from build123d import *

# Parameters (mm, degrees)
PAD_DEPTH       = 10
POCKET_DEPTH    = 6
POCKET001_DEPTH = 6
POCKET002_DEPTH = 11
FILLET_R        = 1
FILLET001_R     = 10
FILLET002_R     = 9
FILLET003_R     = 1


with BuildPart() as part:
    # Sketch → Pad (new body)
    with BuildSketch(Plane.XY):
        Polygon((-65, 10), (-65, 5), (-60, 5), (-60, -5), (-75, -5), (-75, -35), (-50, -35), (-50, -5), (-30, -5), (-30, 0), (-35, 0), (-35, 5), (-30, 5), (-30, 10), (-45, 10), (-45, 5), (-40, 5), (-40, 0), (-55, 0), (-55, 5), (-50, 5), (-50, 10), align=None)
    extrude(amount=PAD_DEPTH)

    # Sketch001 (on Face24 of Pad) → Pocket (cut)
    with BuildSketch(Plane.XY.offset(10)):
        Polygon((0, 15), (-80, 15), (-80, -5), (-60, -5), (-60, -35), (-50, -35), (-50, -5), (0, -5), align=None)
    extrude(amount=-POCKET_DEPTH, mode=Mode.SUBTRACT)

    # Sketch002 (on Face27 of Pocket) → Pocket001 (cut)
    with BuildSketch(Plane.XY.offset(10)):
        Polygon((-80, -8.189183), (-60, -11), (-60, -31), (-80, -28.189183), align=None)
    extrude(amount=-POCKET001_DEPTH, mode=Mode.SUBTRACT)

    # Sketch003 (on Face29 of Pocket001) → Pocket002 (cut)
    with BuildSketch(Plane.XY.offset(10)):
        Polygon((-60, -35), (-80, -32.189183), (-80, -40), (-60, -40), align=None)
    extrude(amount=-POCKET002_DEPTH, mode=Mode.SUBTRACT)

    # Fillet
    fillet_edges = [part.edges().sort_by_distance(p)[0] for p in [
        (-65, 5, 2),
        (-45, 5, 2),
        (-45, 10, 2),
        (-65, 10, 2),
        (-50, 10, 2),
        (-30, 10, 2),
        (-50, 5, 2),
        (-30, 5, 2),
    ]]
    fillet(fillet_edges, radius=FILLET_R)

    # Fillet001
    fillet001_edges = [part.edges().sort_by_distance(p)[0] for p in [
        (-50, -5, 2),
    ]]
    fillet(fillet001_edges, radius=FILLET001_R)

    # Fillet002
    fillet002_edges = [part.edges().sort_by_distance(p)[0] for p in [
        (-50, -35, 2),
    ]]
    fillet(fillet002_edges, radius=FILLET002_R)

    # Fillet003
    fillet003_edges = [part.edges().sort_by_distance(p)[0] for p in [
        (-30, -5, 2),
        (-30, 0, 2),
    ]]
    fillet(fillet003_edges, radius=FILLET003_R)


solid = part.part
The model under review builds one solid part; all positions refer to its coordinate system, in mm. A direction names the side the tool comes from. Give positions to 0.01 mm unless a question says otherwise; leave off trailing zeros. Order: outer loops, then holes, each group sorted by start corner. A loop starts at its lowest first (then second) coordinate and runs counter-clockwise, first axis right, second up. Notation, with made-up numbers: M 8.5,84.25 L 62.5,84.25 A12 ccw 62.5,91.25 Z; hole C 22.25,77 d1. An arc over 180 degrees is marked long. Answer in a Markdown table with one row per item. Add a question column.
1. For pin 1 Ø2 at (y, z) = (-16.5, 3) entering from +X; pin 2 Ø2 at (y, z) = (-30, 3) entering from +X; pin 3 Ø4.5 at (x, z) = (-42, 2.5) entering from -Y, all flat-tipped, find the tip position at first contact; note any pin that passes through.
2. Add section A-A on z = 8.25. State the section outline as (x, y) points, plus the area to 3 significant figures.
3. Machinability: for faces 1 (the flat face through (-60, -33, 7)), 2 (the cylindrical face through (-30.285, 5.301, 2.028)), 3 (the flat face through (-50, 7, 2)), which of the approach directions +Z, -Z, +X, -X, +Y, -Y give a long, thin tool a straight path to every point of the face, cutting with its end or side? Answer none if there is none.
4. Add section B-B on y = 1.5. State the section outline as (x, z) points, plus the area to 3 significant figures.
5. Add section C-C on x = -62.5. State the section outline as (y, z) points, plus the area to 3 significant figures.
6. Mouldability with a two-part tool opening along Y and no side actions: class faces 4 (the flat face through (-45, 8, 2)), 5 (the cylindrical face through (-52.566, -32.294, 2.028)), 6 (the flat face through (-55, 2, 2)) as released by +Y, released by -Y, zero draft, split by the parting line, or undercut.
7. Add section D-D on y = -7. State the section outline as (x, z) points, plus the area to 3 significant figures.
8. To check wall thickness, follow line 1 along X through (y, z) = (1, 0.5); line 2 along Z through (x, y) = (-67, -12.5); line 3 along Y through (x, z) = (-62, 7). State the ranges of each line that lie inside material, in increasing order.
The answers:
| question | item | result |
|---|---|---|
| 1 | pin 1 | x = -50 |
| 1 | pin 2 | x = -50.51 |
| 1 | pin 3 | y = -5.95 |
| 2 | outline | M -75,-32.89 L -60,-35 L -60,-31 L -75,-28.89 Z; M -75,-8.89 L -60,-11 L -60,-5 L -75,-5 Z |
| 2 | area | 134 mm2 |
| 3 | face 1 | +Z, +X, +Y, -Y |
| 3 | face 2 | +Z, -Z, +X |
| 3 | face 3 | +Z, -Z, +Y |
| 4 | outline | M -60,0 L -55,0 L -55,4 L -60,4 Z; M -40,0 L -35,0 L -35,4 L -40,4 Z |
| 4 | area | 40.0 mm2 |
| 5 | outline | M -34.65,0 L -5,0 L -5,10 L -10.65,10 L -10.65,4 L -30.65,4 L -30.65,10 L -34.65,10 Z; M 5,0 L 10,0 L 10,4 L 5,4 Z |
| 5 | area | 196 mm2 |
| 6 | face 4 | zero draft |
| 6 | face 5 | released by -Y |
| 6 | face 6 | undercut |
| 7 | outline | M -75,0 L -46,0 L -46,4 L -60,4 L -60,10 L -75,10 Z |
| 7 | area | 206 mm2 |
| 8 | line 1 | -60 to -55, -40 to -35 |
| 8 | line 2 | 0 to 4 |
| 8 | line 3 | -34.72 to -30.72, -10.72 to -5 |
